Verification items for the finished model (mm, model axes). Face numbers are marked on the shaded views. A direction names the side the tool comes from. Round coordinates to 2 decimals unless told otherwise and drop trailing zeros. Write each loop counter-clockwise with the first axis right and the second up, starting at its lowest first coordinate (ties: lowest second). Pieces come first, ordered by that corner, then holes. Notation, with made-up numbers: (24, 16) - (61, 16) arc R17 ccw to (61, 34) - close; hole circle Ø4 at (84, 63). An arc over 180 degrees is marked (long way). Answer as a JSON object with one key per item and string values. Group by question number.
1) Section check C-C (y = 38). Enter the section's corners in (x, z).
2) Thickness scan on line 1 (X direction, y = 26.55, z = 1.85); line 2 (Y direction, x = 25, z = 3.2); line 3 (Z direction, x = 20, y = 24). Record the ranges inside material, lowest first.
3) Go/stop test with flat-tipped pins: pin 1 Ø6 at (x, z) = (57, -6.5) entering from +Y; pin 2 Ø8 at (x, z) = (53, -7) entering from -Y; pin 3 Ø3 at (y, z) = (41.5, 1) entering from +X; pin 4 Ø4.5 at (y, z) = (37.5, -2.5) entering from -X. Record where each tip stops, or that it passes through.
4) Section check D-D (z = -2.5). Enter the section's corners in (x, y).
5) Section check A-A (x = 25). Enter the section's corners in (y, z) (3 decimals), then the cut area to 3 significant figures.
6) Set-up check for the marked faces 1, 2 and 3: record each of +Z, -Z, +X, -X, +Y, -Y from which the full face is reachable in a straight line by a thin tool's end or side.
7) Section check B-B (x = 51). Enter the section's corners in (y, z).
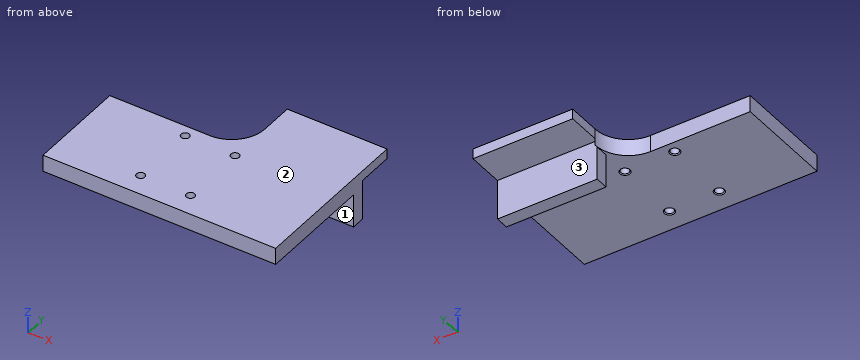
```python
from build123d import *

# Parameters (mm, degrees)
BODY_DEPTH           = 5
LPATTERN1_COUNT      = 2
LPATTERN1_PITCH      = 15
LPATTERN1_COUNT_DIR2 = 2
LPATTERN1_PITCH_DIR2 = 20
SKETCH4_W            = 30
SKETCH4_H            = 2
CUT_EXTRUDE2_DEPTH   = 12
SKETCH5_W            = 30
SKETCH5_H            = 1
BOSS_EXTRUDE3_DEPTH  = 12
SKETCH6_W            = 30
SKETCH6_H            = 10
BOSS_EXTRUDE4_DEPTH  = 3


with BuildPart() as part:
    # Sketch1 → Body (new body)
    with BuildSketch(Plane.XY):
        with BuildLine():
            Line((0, 0), (70, 0))
            Line((70, 0), (70, 50))
            Line((70, 50), (40, 50))
            Line((40, 50), (40, 40))
            ThreePointArc((40, 40), (37.071067812, 32.928932188), (30, 30))
            Line((30, 30), (0, 30))
            Line((0, 30), (0, 0))
        make_face()
    extrude(amount=BODY_DEPTH)

    # Sketch8 → M3x0.5 Tapped Hole1 (revolve, cut)
    with BuildSketch(Plane(origin=(25, 6.55, 5), x_dir=(0, -1, 0), z_dir=(1, 0, 0))):
        Polygon((0, 0), (0, 5), (1.525, 5), (1.25, 4.725), (1.25, 0), align=None)
    m3x0_5_tapped_hole1 = revolve(axis=Axis((25, 6.55, 11.35), (0, 0, -1)), mode=Mode.SUBTRACT)

    # LPattern1: M3x0.5 Tapped Hole1 2 × 2
    with Locations(*[(i * LPATTERN1_PITCH, j * LPATTERN1_PITCH_DIR2, 0) for i in range(LPATTERN1_COUNT) for j in range(LPATTERN1_COUNT_DIR2) if (i, j) != (0, 0)]):
        add(m3x0_5_tapped_hole1, mode=Mode.SUBTRACT)

    # Sketch4 → Cut-Extrude2 (cut)
    with BuildSketch(Plane(origin=(0, 50, 0), x_dir=(1, 0, 0), z_dir=(0, 1, 0))):
        with Locations((55, -1)):
            Rectangle(SKETCH4_W, SKETCH4_H)
    extrude(amount=-CUT_EXTRUDE2_DEPTH, mode=Mode.SUBTRACT)

    # Sketch5 → Boss-Extrude3 (add)
    with BuildSketch(Plane(origin=(0, 0, 2), x_dir=(-1, 0, 0), z_dir=(0, 0, -1))):
        with Locations((-55, 38.5)):
            Rectangle(SKETCH5_W, SKETCH5_H)
    extrude(amount=BOSS_EXTRUDE3_DEPTH)

    # Sketch6 → Boss-Extrude4 (add)
    with BuildSketch(Plane.XZ.offset(-38)):
        with Locations((55, -5)):
            Rectangle(SKETCH6_W, SKETCH6_H)
    extrude(amount=BOSS_EXTRUDE4_DEPTH)


solid = part.part
```
Returned:
{
 "1": {"outline": "(39.8, 0) - (40, 0) - (40, -10) - (70, -10) - (70, 5) - (39.8, 5) - close"},
 "2": {"line 1": "0 to 23.75, 26.25 to 38.75, 41.25 to 70", "line 2": "0 to 5.3, 7.8 to 25.3, 27.8 to 30", "line 3": "0 to 5"},
 "3": {"pin 1": "y = 39", "pin 2": "y = 35", "pin 3": "x = 70", "pin 4": "x = 40"},
 "4": {"outline": "(40, 35) - (70, 35) - (70, 39) - (40, 39) - close"},
 "5": {"outline": "(0, 0) - (5.025, 0) - (5.3, 0.275) - (5.3, 5) - (0, 5) - close; (7.8, 0.275) - (8.075, 0) - (25.025, 0) - (25.3, 0.275) - (25.3, 5) - (7.8, 5) - close; (27.8, 0.275) - (28.075, 0) - (30, 0) - (30, 5) - (27.8, 5) - close", "area": "125 mm2"},
 "6": {"face 1": "-Z, +X, -X, -Y", "face 2": "+Z, +X, -X, +Y, -Y", "face 3": "-Z, +X, +Y"},
 "7": {"outline": "(0, 0) - (35, 0) - (35, -10) - (39, -10) - (39, 2) - (50, 2) - (50, 5) - (0, 5) - close"}
}
